The drawing under review shows one solid part. Ordinate dimensions are in mm from its lowest x, y, z. Round coordinates to 2 decimals unless told otherwise and drop trailing zeros. Order: outer loops, then holes, each group sorted by start corner. A loop starts at its lowest first (then second) coordinate and runs counter-clockwise, first axis right, second up. Notation, with made-up numbers: (75.25, 33) - (121.25, 33) arc R12 cw to (121.25, 42) - close; hole circle Ø2 at (46, 17.25). An arc over 180 degrees is marked (long way). One line per question, with ' | ' between items.
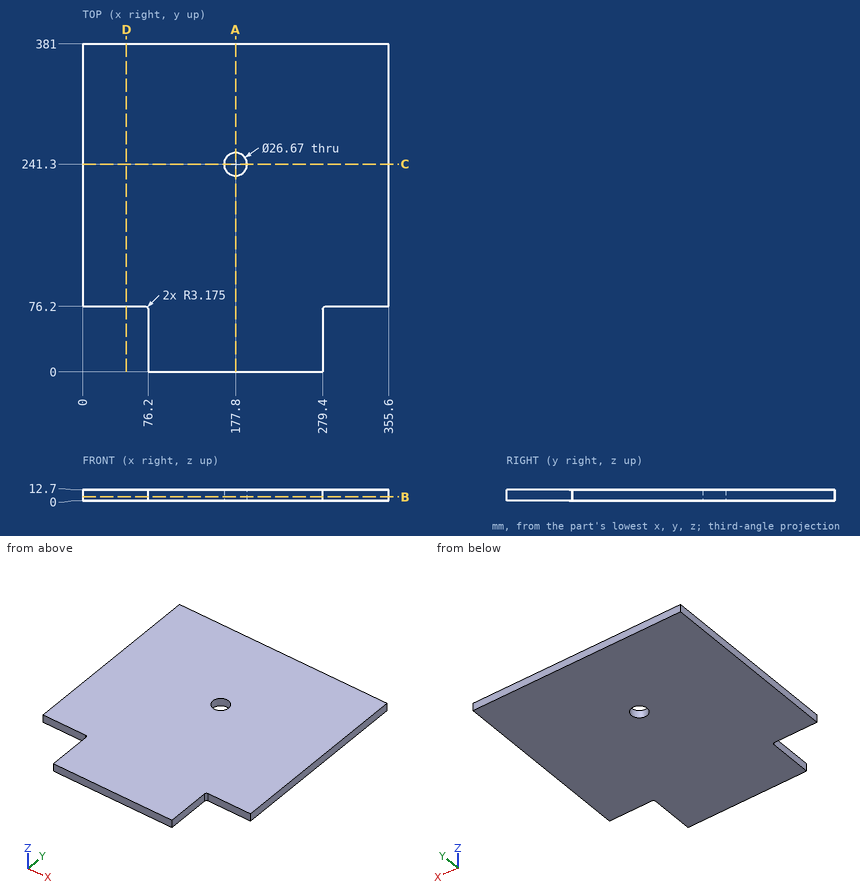
(1) We need section D-D on x = 51. State the section outline as (y, z) points.
Output values:
outline: (76.2, 0) - (381, 0) - (381, 12.7) - (76.2, 12.7) - close
(2) For probe 1 along Y at (x, z) = (177.8, 8.25) (3 decimals); probe 2 along Y at (x, z) = (286.5, 10.5); probe 3 along X at (y, z) = (34, 6.75), list the stretches that pass through material, from the lowest coordinate up. Write a range as [from, to].
Output values:
probe 1: [0, 227.965], [254.635, 381] | probe 2: [76.2, 381] | probe 3: [76.2, 279.4]
(3) We need section B-B on z = 4.5. State the section outline as (x, y) points (3 decimals), plus the area to 3 significant figures.
Output values:
outline: (0, 76.2) - (73.025, 76.2) arc R3.175 cw to (76.2, 73.025) - (76.2, 0) - (279.4, 0) - (279.4, 73.025) arc R3.175 cw to (282.575, 76.2) - (355.6, 76.2) - (355.6, 381) - (0, 381) - close; hole circle Ø26.67 at (177.8, 241.3) | area: 123,000 mm^2
(4) Insertion check: pin 1 (5 mm diameter, centred on y = 45, z = 5, fed in from -X); pin 2 (5 mm diameter, centred on x = 43, y = 157.5, fed in from -Z); pin 3 (6.5 mm diameter, centred on y = 21, z = 9.5, fed in from +X); pin 4 (6.5 mm diameter, centred on x = 49.5, z = 4, fed in from -Y). Each pin has a flat end and moves straight along its axis. Give the tip position at first contact, or say it passes through.
Output values:
pin 1: x = 76.2 | pin 2: z = 0 | pin 3: x = 279.4 | pin 4: y = 76.2
(5) We need section C-C on y = 241.3. State the section outline as (x, z) points (3 decimals), plus the area to 3 significant figures.
Output values:
outline: (0, 0) - (164.465, 0) - (164.465, 12.7) - (0, 12.7) - close; (191.135, 0) - (355.6, 0) - (355.6, 12.7) - (191.135, 12.7) - close | area: 4,180 mm^2
(6) We need section A-A on x = 177.8. State the section outline as (y, z) points (3 decimals), plus the area to 3 significant figures.
Output values:
outline: (0, 0) - (227.965, 0) - (227.965, 12.7) - (0, 12.7) - close; (254.635, 0) - (381, 0) - (381, 12.7) - (254.635, 12.7) - close | area: 4,500 mm^2
